The listing builds one solid part. Answer for the finished solid, in the listing's coordinates (mm). A direction names the side the tool comes from. Coordinates: 2 decimals unless noted, no trailing zeros. Order: outer loops, then holes, each group sorted by start corner. A loop starts at its lowest first (then second) coordinate and runs counter-clockwise, first axis right, second up. Notation, with made-up numbers: (-8.75, 25) - (40.25, 25) arc R11 ccw to (40.25, 36) - close; hole circle Ø8 at (27, 28.5). An arc over 180 degrees is marked (long way). One line per item, written item: value. Start each with the question number.
```python
from build123d import *

# Parameters (mm, degrees)
BOSS_EXTRUDE1_DEPTH = 4
FILLET2_R           = 2
CUT_EXTRUDE1_REACH  = 194.09
SKETCH2_R           = 1.6
SKETCH3_R           = 4
SKETCH3_R_2         = 1.6
BOSS_EXTRUDE2_DEPTH = 4


with BuildPart() as part:
    # Sketch1 → Boss-Extrude1 (new body)
    with BuildSketch(Plane(origin=(0, 0, 0), x_dir=(1, 0, 0), z_dir=(0, 1, 0))):
        with BuildLine():
            Line((-22.921559452, -129.994623398), (-23.78980034, -134.918662163))
            ThreePointArc((-23.78980034, -134.918662163), (-137, 0), (-23.78980034, 134.918662163))
            Line((-23.78980034, 134.918662163), (-22.921559452, 129.994623398))
            ThreePointArc((-22.921559452, 129.994623398), (-132, 0), (-22.921559452, -129.994623398))
        make_face()
    extrude(amount=BOSS_EXTRUDE1_DEPTH)

    # Fillet2
    fillet2_edges = [part.edges().sort_by_distance(p)[0] for p in [
        (-23.78980034, 2, -134.918662163),
        (-23.78980034, 2, 134.918662163),
        (-22.921559452, 2, 129.994623398),
        (-22.921559452, 2, -129.994623398),
    ]]
    fillet(fillet2_edges, radius=FILLET2_R)

    # Sketch2 → Cut-Extrude1 (cut, up to next)
    with BuildSketch(Plane(origin=(0, 4, 0), x_dir=(1, 0, 0), z_dir=(0, 1, 0)), mode=Mode.PRIVATE) as cut_extrude1_sk1:
        with Locations(Location((-66.779143443, 116.751, 0), (0, 0, 270))):
            Circle(SKETCH2_R)
    cut_extrude1_tool1 = extrude(cut_extrude1_sk1.sketch, amount=-CUT_EXTRUDE1_REACH, mode=Mode.PRIVATE) & part.part
    # Sketch2 → Cut-Extrude1 (cut, up to next)
    with BuildSketch(Plane(origin=(0, 4, 0), x_dir=(1, 0, 0), z_dir=(0, 1, 0)), mode=Mode.PRIVATE) as cut_extrude1_sk2:
        with Locations(Location((-134.5, 0, 0), (0, 0, 270))):
            Circle(SKETCH2_R)
    cut_extrude1_tool2 = extrude(cut_extrude1_sk2.sketch, amount=-CUT_EXTRUDE1_REACH, mode=Mode.PRIVATE) & part.part
    # Sketch2 → Cut-Extrude1 (cut, up to next)
    with BuildSketch(Plane(origin=(0, 4, 0), x_dir=(1, 0, 0), z_dir=(0, 1, 0)), mode=Mode.PRIVATE) as cut_extrude1_sk3:
        with Locations(Location((-66.779143443, -116.751, 0), (0, 0, 270))):
            Circle(SKETCH2_R)
    cut_extrude1_tool3 = extrude(cut_extrude1_sk3.sketch, amount=-CUT_EXTRUDE1_REACH, mode=Mode.PRIVATE) & part.part
    add(cut_extrude1_tool1.solids().sort_by_distance((-66.779143, 4, -116.751))[0], mode=Mode.SUBTRACT)
    add(cut_extrude1_tool2.solids().sort_by_distance((-134.5, 4, 0))[0], mode=Mode.SUBTRACT)
    add(cut_extrude1_tool3.solids().sort_by_distance((-66.779143, 4, 116.751))[0], mode=Mode.SUBTRACT)

    # Sketch3 → Boss-Extrude2 (add)
    # profile 1 of 3: a face of its own
    with BuildSketch(Plane(origin=(0, 4, 0), x_dir=(1, 0, 0), z_dir=(0, 1, 0))):
        with Locations((-66.779143443, -116.751)):
            Circle(SKETCH3_R)
        with Locations(Location((-66.779143443, -116.751, 0), (0, 0, 270))):
            Circle(SKETCH3_R_2, mode=Mode.SUBTRACT)
    # profile 2 of 3: a face of its own
    with BuildSketch(Plane(origin=(0, 4, 0), x_dir=(1, 0, 0), z_dir=(0, 1, 0))):
        with Locations((-134.5, 0)):
            Circle(SKETCH3_R)
        with Locations(Location((-134.5, 0, 0), (0, 0, 270))):
            Circle(SKETCH3_R_2, mode=Mode.SUBTRACT)
    # profile 3 of 3: a face of its own
    with BuildSketch(Plane(origin=(0, 4, 0), x_dir=(1, 0, 0), z_dir=(0, 1, 0))):
        with Locations((-66.779143443, 116.751)):
            Circle(SKETCH3_R)
        with Locations(Location((-66.779143443, 116.751, 0), (0, 0, 270))):
            Circle(SKETCH3_R_2, mode=Mode.SUBTRACT)
    extrude(amount=-BOSS_EXTRUDE2_DEPTH)


solid = part.part
```
(1) Flat-ended cylindrical pins translate along their axes: pin 1 Ø1 at (x, y) = (-103.5, 2) entering from +Z; pin 2 Ø2 at (x, y) = (-68, 1) entering from +Z; pin 3 Ø2.5 at (x, z) = (-134.5, 0) entering from +Y; pin 4 Ø2 at (x, y) = (-116, 2) entering from +Z. Find the tip coordinate at first contact, or state that the pin passes through.
(2) The part is cut by section A-A on x = -124. Determine the outline of the cut face in (y, z).
(3) For a pull along Z with two mould halves and no side action, classify faces 3 (the face through (-118.99, 1.97, -67.9)), 4 (the face through (-113.713, 1.972, -67.032)), 5 (the face through (-132, 4, -1)) as pulls with the +Z half, pulls with the -Z half, needs draft (parallel to the pull), parting line crosses it, or undercut.
(4) The part is cut by section C-C on x = -76.5. Determine the outline of the cut face in (y, z), plus the area to 3 significant figures.
(5) For faces 1 (the face through (-118.02, 1.97, 69.57)), 2 (the face through (-44.101, 1.972, -124.415)), determine the directions among +Z, -Z, +X, -X, +Y, -Y from which every point of the face is accessible in a straight line to the end or side of a thin tool.
(6) Consider probe 1 along Z at (x, y) = (-103.5, 1); probe 2 along Z at (x, y) = (-67.5, 3); probe 3 along Z at (x, y) = (-85, 2.8). Determine where each line is inside the solid, lowest interval first.
(7) The part is cut by section B-B on y = 1.4. Determine the outline of the cut face in (x, z), plus the area to 3 significant figures.
(8) The part is cut by section D-D on z = -51. Determine the outline of the cut face in (x, y).
Completed:
1. pin 1: stops at z = 90.33
1. pin 2: stops at z = 120.74
1. pin 3: passes through
1. pin 4: stops at z = 74.46
2. outline: (0, -58.25) - (4, -58.25) - (4, -45.25) - (0, -45.25) - close; (0, 45.25) - (4, 45.25) - (4, 58.25) - (0, 58.25) - close
3. face 3: pulls with the -Z half
3. face 4: undercut
3. face 5: needs draft
4. outline: (0, -113.65) - (4, -113.65) - (4, -107.57) - (0, -107.57) - close; (0, 107.57) - (4, 107.57) - (4, 113.65) - (0, 113.65) - close
4. area: 48.6 mm2
5. face 1: +Z, -X, +Y, -Y
5. face 2: +X, +Y, -Y
6. probe 1: z = -89.76 to -81.93, 81.93 to 89.76
6. probe 2: z = -120.69 to -118.18, -115.32 to -112.82, 112.82 to 115.32, 118.18 to 120.69
6. probe 3: z = -107.44 to -100.99, 100.99 to 107.44
7. outline: (-136.96, -3.15) arc R137 ccw to (-70.74, -117.33) arc R4 ccw to (-65.27, -120.45) arc R137 ccw to (-25.79, -134.55) arc R2 ccw to (-23.44, -132.93) - (-23.27, -131.95) arc R2 ccw to (-24.86, -129.64) arc R132 cw to (-62.83, -116.09) arc R4 ccw to (-68.2, -113.01) arc R132 cw to (-131.96, -3.09) arc R4 ccw to (-131.96, 3.09) arc R132 cw to (-68.2, 113.01) arc R4 ccw to (-62.83, 116.09) arc R132 cw to (-24.86, 129.64) arc R2 ccw to (-23.27, 131.95) - (-23.44, 132.93) arc R2 ccw to (-25.79, 134.55) arc R137 ccw to (-65.27, 120.45) arc R4 ccw to (-70.74, 117.33) arc R137 ccw to (-136.96, 3.15) arc R4 ccw to start; hole circle Ø3.2 at (-134.5, 0); hole circle Ø3.2 at (-66.78, -116.75); hole circle Ø3.2 at (-66.78, 116.75)
7. area: 1,890 mm2
8. outline: (-127.15, 0) - (-121.75, 0) - (-121.75, 4) - (-127.15, 4) - close
